Read the model definition and answer for the solid it produces. Units are mm, in the model's axes. Coordinates: 2 decimals unless noted, no trailing zeros. Order: outer loops, then holes, each group sorted by start corner. A loop starts at its lowest first (then second) coordinate and runs counter-clockwise, first axis right, second up. Notation, with made-up numbers: (64, 29.5) - (82, 29.5) arc R17 ccw to (82, 39.5) - close; hole circle Ø5 at (-7, 14.25). An arc over 180 degrees is marked (long way). Use one line per item in the form item = value.
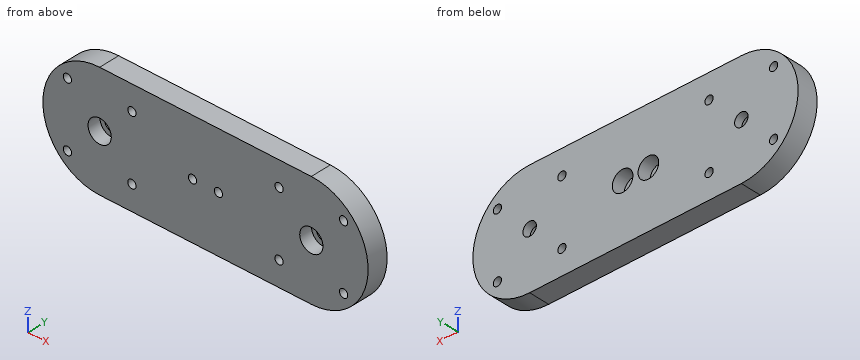
```python
from build123d import *

# Parameters (mm, degrees)
SKETCH_1_R          = 2.6
SKETCH_1_R_2        = 1.6
EXTRUDE_1_DEPTH     = 8
SKETCH_2_R          = 4.5
CUT_EXTRUDE_1_DEPTH = 5
SKETCH_3_R          = 4
CUT_EXTRUDE_2_DEPTH = 5


with BuildPart() as part:
    # 草图1 → 凸台-拉伸1 (new body)
    with BuildSketch(Plane(origin=(0, 0, 0), x_dir=(1, 0, 0), z_dir=(0, 1, 0))):
        with BuildLine():
            Line((0, 22), (82, 22))
            ThreePointArc((82, 22), (104, 0), (82, -22))
            Line((82, -22), (0, -22))
            ThreePointArc((0, -22), (-22, 0), (0, 22))
        make_face()
        with Locations(Location((0, 0, 0), (0, 0, 270))):
            Circle(SKETCH_1_R, mode=Mode.SUBTRACT)
        with Locations(Location((82, 0, 0), (0, 0, 90))):
            Circle(SKETCH_1_R, mode=Mode.SUBTRACT)
        with Locations(Location((12.5, 12.5, 0), (0, 0, 270))):
            Circle(SKETCH_1_R_2, mode=Mode.SUBTRACT)
        with Locations(Location((-12.5, 12.5, 0), (0, 0, 90))):
            Circle(SKETCH_1_R_2, mode=Mode.SUBTRACT)
        with Locations(Location((12.5, -12.5, 0), (0, 0, 90))):
            Circle(SKETCH_1_R_2, mode=Mode.SUBTRACT)
        with Locations(Location((-12.5, -12.5, 0), (0, 0, 270))):
            Circle(SKETCH_1_R_2, mode=Mode.SUBTRACT)
        with Locations(Location((94.5, -12.5, 0), (0, 0, 90))):
            Circle(SKETCH_1_R_2, mode=Mode.SUBTRACT)
        with Locations(Location((69.5, -12.5, 0), (0, 0, 270))):
            Circle(SKETCH_1_R_2, mode=Mode.SUBTRACT)
        with Locations(Location((69.5, 12.5, 0), (0, 0, 90))):
            Circle(SKETCH_1_R_2, mode=Mode.SUBTRACT)
        with Locations(Location((94.5, 12.5, 0), (0, 0, 270))):
            Circle(SKETCH_1_R_2, mode=Mode.SUBTRACT)
        with Locations(Location((36, 0, 0), (0, 0, 270))):
            Circle(SKETCH_1_R_2, mode=Mode.SUBTRACT)
        with Locations(Location((46, 0, 0), (0, 0, 90))):
            Circle(SKETCH_1_R_2, mode=Mode.SUBTRACT)
    extrude(amount=EXTRUDE_1_DEPTH)

    # 草图2 → 切除-拉伸1 (cut)
    with BuildSketch(Plane(origin=(0, 0, 0), x_dir=(-1, 0, 0), z_dir=(0, -1, 0))):
        with Locations(Location((0, 0, 0), (0, 0, 90))):
            Circle(SKETCH_2_R)
        with Locations(Location((-82, 0, 0), (0, 0, 90))):
            Circle(SKETCH_2_R)
    extrude(amount=-CUT_EXTRUDE_1_DEPTH, mode=Mode.SUBTRACT)

    # 草图3 → 切除-拉伸2 (cut)
    with BuildSketch(Plane(origin=(0, 8, 0), x_dir=(1, 0, 0), z_dir=(0, 1, 0))):
        with Locations(Location((36, 0, 0), (0, 0, 270))):
            Circle(SKETCH_3_R)
        with Locations(Location((46, 0, 0), (0, 0, 270))):
            Circle(SKETCH_3_R)
    extrude(amount=-CUT_EXTRUDE_2_DEPTH, mode=Mode.SUBTRACT)


solid = part.part
```
(1) Section A-A, the plane x = 12.5 is taken. Write down the section's boundary in (y, z).
Answer list:
outline = (0, -22) - (8, -22) - (8, -14.1) - (0, -14.1) - close; (0, -10.9) - (8, -10.9) - (8, 10.9) - (0, 10.9) - close; (0, 14.1) - (8, 14.1) - (8, 22) - (0, 22) - close
(2) Straight lines are drawn through the part: L1, parallel to X at y = 7.3, z = 0; L2, parallel to X at y = 1.15, z = 0; L3, parallel to Z at x = 93.5, y = 7.75 (3 decimals). For each, find the intervals that lie inside material, in ascending order.
Answer list:
L1 = -22 to -2.6, 2.6 to 32, 40 to 42, 50 to 79.4, 84.6 to 104
L2 = -22 to -4.5, 4.5 to 34.4, 37.6 to 44.4, 47.6 to 77.5, 86.5 to 104
L3 = -18.755 to -13.749, -11.251 to 11.251, 13.749 to 18.755
(3) Section B-B, the plane y = 6.25 is taken. State how many separate pieces and enclosed holes the cut face has, then the cut area to 3 significant figures.
Answer list:
separate_pieces = 1
enclosed_holes = 12
area = 4,920 mm2
(4) Section C-C, the plane x = 46 is taken. Write down the section's boundary in (y, z).
Answer list:
outline = (0, -22) - (8, -22) - (8, -4) - (3, -4) - (3, -1.6) - (0, -1.6) - close; (0, 1.6) - (3, 1.6) - (3, 4) - (8, 4) - (8, 22) - (0, 22) - close
(5) Given pin 1 Ø10.5 at (x, z) = (46, 0) entering from +Y; pin 2 Ø5.5 at (x, z) = (0, 0) entering from -Y; pin 3 Ø4 at (x, y) = (-3, 7) entering from +Z; pin 4 Ø4 at (y, z) = (1.5, -1.5) entering from +X, each flat-ended and moving along its own axis, determine where each tip first touches the part or whether it passes through.
Answer list:
pin_1 = 8
pin_2 = 5
pin_3 = 21.98
pin_4 = 104
